Geometry: final body of the model. Coordinates: model frame, mm. Coordinates: 2 decimals unless noted, no trailing zeros. Put each result on its own line as item: value.
```python
from build123d import *

# Parameters (mm, degrees)
SKETCH1_W           = 43.5
SKETCH1_H           = 43.5
SKETCH1_R           = 1.5
BOSS_EXTRUDE1_DEPTH = 1.5
CUT_EXTRUDE1_START  = -0.0001
SKETCH2_R           = 2.5
SKETCH2_R_2         = 1.5
CUT_EXTRUDE1_DEPTH  = 0.0001
SKETCH3_R           = 2.5
SKETCH3_R_2         = 1.5
CUT_EXTRUDE2_DEPTH  = 0.002
SKETCH4_W           = 7
SKETCH4_H           = 0.5
CUT_EXTRUDE4_DEPTH  = 0.0001
SKETCH6_W           = 8
SKETCH6_H           = 15
SKETCH6_W_2         = 10
SKETCH6_H_2         = 8
CUT_EXTRUDE5_DEPTH  = 0.0001
SKETCH8_R           = 4
CUT_EXTRUDE6_DEPTH  = 0.0001
SKETCH9_W           = 14.5
SKETCH9_H           = 4
CUT_EXTRUDE7_DEPTH  = 0.0001
SKETCH10_W          = 5
SKETCH10_H          = 15.24
CUT_EXTRUDE8_DEPTH  = 0.0001
SKETCH11_R          = 4
SKETCH11_W          = 14.5
SKETCH11_H          = 4
CUT_EXTRUDE9_DEPTH  = 0.0001
CUT_EXTRUDE10_DEPTH = 0.0001
SKETCH13_W          = 6.9
SKETCH13_H          = 10
CUT_EXTRUDE11_DEPTH = 0.0001


with BuildPart() as part:
    # Sketch1 → Boss-Extrude1 (new body)
    with BuildSketch(Plane.XY):
        Rectangle(SKETCH1_W, SKETCH1_H)
        with Locations((-18.25, 18.25)):
            Circle(SKETCH1_R, mode=Mode.SUBTRACT)
        with Locations((18.25, 18.25)):
            Circle(SKETCH1_R, mode=Mode.SUBTRACT)
        with Locations((18.25, -18.25)):
            Circle(SKETCH1_R, mode=Mode.SUBTRACT)
        with Locations((-18.25, -18.25)):
            Circle(SKETCH1_R, mode=Mode.SUBTRACT)
    extrude(amount=BOSS_EXTRUDE1_DEPTH)

    # Sketch2 → Cut-Extrude1 (cut)
    # profile 1 of 4: a face of its own
    with BuildSketch(Plane.XY.offset(1.5).offset(CUT_EXTRUDE1_START)):
        with Locations((-18.25, 18.25)):
            Circle(SKETCH2_R)
        with Locations((-18.25, 18.25)):
            Circle(SKETCH2_R_2, mode=Mode.SUBTRACT)
    # profile 2 of 4: a face of its own
    with BuildSketch(Plane.XY.offset(1.5).offset(CUT_EXTRUDE1_START)):
        with Locations((18.758938316, 18.758938316)):
            Circle(SKETCH2_R)
        with Locations((18.758938316, 18.758938316)):
            Circle(SKETCH2_R_2, mode=Mode.SUBTRACT)
    # profile 3 of 4: a face of its own
    with BuildSketch(Plane.XY.offset(1.5).offset(CUT_EXTRUDE1_START)):
        with Locations((19.267876631, -18.25)):
            Circle(SKETCH2_R)
        with Locations((19.267876631, -18.25)):
            Circle(SKETCH2_R_2, mode=Mode.SUBTRACT)
    # profile 4 of 4: a face of its own
    with BuildSketch(Plane.XY.offset(1.5).offset(CUT_EXTRUDE1_START)):
        with Locations((-17.741061684, -18.758938316)):
            Circle(SKETCH2_R)
        with Locations((-17.741061684, -18.758938316)):
            Circle(SKETCH2_R_2, mode=Mode.SUBTRACT)
    extrude(amount=CUT_EXTRUDE1_DEPTH, mode=Mode.SUBTRACT)

    # Sketch3 → Cut-Extrude2 (cut)
    # profile 1 of 4: a face of its own
    with BuildSketch(Plane(origin=(0, 0, 0), x_dir=(-1, 0, 0), z_dir=(0, 0, -1))):
        with Locations((-18.25, -18.25)):
            Circle(SKETCH3_R)
        with Locations((-18.25, -18.25)):
            Circle(SKETCH3_R_2, mode=Mode.SUBTRACT)
    # profile 2 of 4: a face of its own
    with BuildSketch(Plane(origin=(0, 0, 0), x_dir=(-1, 0, 0), z_dir=(0, 0, -1))):
        with Locations(Location((-18.758938316, 18.758938316, 0), (0, 0, 180))):
            Circle(SKETCH3_R)
        with Locations((-18.758938316, 18.758938316)):
            Circle(SKETCH3_R_2, mode=Mode.SUBTRACT)
    # profile 3 of 4: a face of its own
    with BuildSketch(Plane(origin=(0, 0, 0), x_dir=(-1, 0, 0), z_dir=(0, 0, -1))):
        with Locations((18.25, 19.267876631)):
            Circle(SKETCH3_R)
        with Locations((18.25, 19.267876631)):
            Circle(SKETCH3_R_2, mode=Mode.SUBTRACT)
    # profile 4 of 4: a face of its own
    with BuildSketch(Plane(origin=(0, 0, 0), x_dir=(-1, 0, 0), z_dir=(0, 0, -1))):
        with Locations((18.758938316, -17.741061684)):
            Circle(SKETCH3_R)
        with Locations((18.758938316, -17.741061684)):
            Circle(SKETCH3_R_2, mode=Mode.SUBTRACT)
    extrude(amount=-CUT_EXTRUDE2_DEPTH, mode=Mode.SUBTRACT)

    # Sketch4 → Cut-Extrude4 (cut)
    with BuildSketch(Plane.XY.offset(1.5)):
        Polygon((14.95, 11), (21.65, 11), (21.65, 11.5), (12.65, 11.5), (12.65, 11), (12.65, -11), (12.65, -11.5), (21.65, -11.5), (21.65, -11), (14.95, -11), (14.95, -7), (21.65, -7), (21.65, -6.5), (13.55, -6.5), (13.55, -2.5), (21.65, -2.5), (21.65, -2), (14.95, -2), (14.95, 2), (21.65, 2), (21.65, 2.5), (13.55, 2.5), (13.55, 6.5), (21.65, 6.5), (21.65, 7), (14.95, 7), align=None)
        with Locations((9.15, 11.25)):
            Rectangle(SKETCH4_W, SKETCH4_H)
        with Locations((9.15, -11.25)):
            Rectangle(SKETCH4_W, SKETCH4_H)
    extrude(amount=-CUT_EXTRUDE4_DEPTH, mode=Mode.SUBTRACT)

    # Sketch6 → Cut-Extrude5 (cut)
    with BuildSketch(Plane.XY.offset(1.5)):
        with Locations((-17.15, 7.65)):
            Rectangle(SKETCH6_W, SKETCH6_H)
        with Locations((-7.55, 17.15)):
            Rectangle(SKETCH6_W_2, SKETCH6_H_2)
        with Locations((-7.55, -17.15)):
            Rectangle(SKETCH6_W_2, SKETCH6_H_2)
    extrude(amount=-CUT_EXTRUDE5_DEPTH, mode=Mode.SUBTRACT)

    # Sketch8 → Cut-Extrude6 (cut)
    with BuildSketch(Plane.XY.offset(1.5)):
        Polygon((-0.05, 7.98), (-2.52, 10.45), (-5.88, 10.45), (-8.35, 7.98), (-8.35, 2.15), (-0.05, 2.15), align=None)
        with Locations((-4.2, 6.3)):
            Circle(SKETCH8_R, mode=Mode.SUBTRACT)
    extrude(amount=-CUT_EXTRUDE6_DEPTH, mode=Mode.SUBTRACT)

    # Sketch9 → Cut-Extrude7 (cut)
    with BuildSketch(Plane.XY.offset(1.5)):
        with Locations((7.5, 18.05)):
            Rectangle(SKETCH9_W, SKETCH9_H)
    extrude(amount=-CUT_EXTRUDE7_DEPTH, mode=Mode.SUBTRACT)

    # Sketch10 → Cut-Extrude8 (cut)
    with BuildSketch(Plane.XY.offset(1.5)):
        with Locations((-17.85, -8.33)):
            Rectangle(SKETCH10_W, SKETCH10_H)
    extrude(amount=-CUT_EXTRUDE8_DEPTH, mode=Mode.SUBTRACT)

    # Sketch11 → Cut-Extrude9 (cut)
    # profile 1 of 2: a face of its own
    with BuildSketch(Plane.XY.offset(1.5)):
        Polygon((-9.42, -2.55), (-12.78, -2.55), (-15.25, -5.02), (-15.25, -10.85), (-6.95, -10.85), (-6.95, -5.02), align=None)
        with Locations((-11.1, -6.7)):
            Circle(SKETCH11_R, mode=Mode.SUBTRACT)
    # profile 2 of 2: a face of its own
    with BuildSketch(Plane.XY.offset(1.5)):
        with Locations((7.5, -18.05)):
            Rectangle(SKETCH11_W, SKETCH11_H)
    extrude(amount=-CUT_EXTRUDE9_DEPTH, mode=Mode.SUBTRACT)

    # Sketch12 → Cut-Extrude10 (cut)
    with BuildSketch(Plane.XY.offset(1.5)):
        Polygon((-9.81, 11.04), (-10.52, 11.75), (-11.64, 11.75), (-12.35, 11.04), (-12.35, 7.46), (-11.64, 6.75), (-10.52, 6.75), (-9.81, 7.46), align=None)
    extrude(amount=-CUT_EXTRUDE10_DEPTH, mode=Mode.SUBTRACT)

    # Sketch13 → Cut-Extrude11 (cut)
    with BuildSketch(Plane.XY.offset(1.5)):
        with Locations((-2.5, -5.75)):
            Rectangle(SKETCH13_W, SKETCH13_H)
    extrude(amount=-CUT_EXTRUDE11_DEPTH, mode=Mode.SUBTRACT)


solid = part.part
```
1. Section query A-A (y = 18.25). Count the separate pieces of the cut face and the enclosed holes in it, then the cut area to 3 significant figures.
Answer below:
separate pieces: 3
enclosed holes: 0
area: 56.2 mm²
2. Mould query, pull axis Y, two halves, no side actions, for faces 1 (the flat face through (0, 21.75, 1)), 2 (the cylindrical face through (-19.75, -18.18, 0.74)), 3 (the flat face through (20, 20, 0.002)). Classes: +Y half, -Y half, draft (parallel to the pull), parting line (faces both ways), or undercut.
Answer below:
face 1: +Y half
face 2: undercut
face 3: draft
3. Ray query, probe 1 along Y at (x, z) = (18.25, 0.65); probe 2 along Y at (x, z) = (17.5, 1.1). Return the intervals inside material, ascending. Write a range as from..to.
Answer below:
probe 1: y = -21.75..-19.75, -16.75..16.75, 19.75..21.75
probe 2: y = -21.75..-19.55, -16.95..16.95, 19.55..21.75
